Autodesk Inventor part; units mm, degrees
ref_plane "YZ Plane" through (0, 0, 0) normal (1, 0, 0) x (0, 1, 0)
ref_plane "XZ Plane" through (0, 0, 0) normal (0, 1, 0) x (-1, 0, 0)
ref_plane "XY Plane" through (0, 0, 0) normal (0, 0, 1) x (1, 0, 0)
sketch "bed" plane through (0, 0, 0) normal (0, 1, 0) x (-1, 0, 0)
  line L0 (59.3441, 94.0804) -> (59.3441, 91.0804)
  line L1 (59.3441, 91.0804) -> (91.3441, 91.0804)
  line L2 (-18.6559, 94.0804) -> (-18.6559, 91.0804)
  line L3 (-18.6559, 91.0804) -> (19.3441, 91.0804)
  line L4 (19.3441, 91.0804) -> (19.3441, 94.0804)
  line L5 (-18.6559, 94.0804) -> (-58.6559, 94.0804)
  line L6 (-58.6559, 94.0804) -> (-58.6559, 91.0804)
  line L7 (59.3441, 94.0804) -> (19.3441, 94.0804)
  line L8 (-58.6559, 91.0804) -> (-90.6559, 91.0804)
  line L9 (59.3441, -93.9196) -> (59.3441, -90.9196)
  line L10 (59.3441, -90.9196) -> (91.3441, -90.9196)
  line L11 (-18.6559, -93.9196) -> (-18.6559, -90.9196)
  line L12 (-18.6559, -90.9196) -> (19.3441, -90.9196)
  line L13 (-58.6559, -93.9196) -> (-58.6559, -90.9196)
  line L14 (59.3441, -93.9196) -> (19.3441, -93.9196)
  line L15 (-18.6559, -93.9196) -> (-58.6559, -93.9196)
  line L16 (-58.6559, -90.9196) -> (-90.6559, -90.9196)
  line L17 (94.3441, 59.0804) -> (91.3441, 59.0804)
  line L18 (94.3441, 59.0804) -> (94.3441, 19.0804)
  line L19 (91.3441, -18.9196) -> (91.3441, 19.0804)
  line L20 (94.3441, -18.9196) -> (91.3441, -18.9196)
  line L21 (94.3441, -58.9196) -> (91.3441, -58.9196)
  line L22 (94.3441, -18.9196) -> (94.3441, -58.9196)
  line L23 (91.3441, 59.0804) -> (91.3441, 91.0804)
  line L24 (91.3441, -58.9196) -> (91.3441, -90.9196)
  line L25 (84.2181, 86.0804) -> (-83.7819, 86.0804)
  line L26 (-85.7819, 84.0804) -> (-85.7819, -83.9196)
  line L27 (-83.7819, -85.9196) -> (84.2181, -85.9196)
  line L28 (86.2181, -83.9196) -> (86.2181, 84.0804)
  arc A0 (86.2181, 84.0804) -> (84.2181, 86.0804) centre (84.2181, 84.0804) ccw
  arc A1 (84.2181, -85.9196) -> (86.2181, -83.9196) centre (84.2181, -83.9196) ccw
  arc A2 (-85.7819, -83.9196) -> (-83.7819, -85.9196) centre (-83.7819, -83.9196) ccw
  arc A3 (-83.7819, 86.0804) -> (-85.7819, 84.0804) centre (-83.7819, 84.0804) ccw
  line L29 (-93.6559, -18.9196) -> (-93.6559, -58.9196)
  line L30 (-93.6559, -58.9196) -> (-90.6559, -58.9196)
  line L31 (-93.6559, -18.9196) -> (-90.6559, -18.9196)
  line L32 (-90.6559, -18.9196) -> (-90.6559, 19.0804)
  line L33 (-90.6559, 19.0804) -> (-93.6559, 19.0804)
  line L34 (-93.6559, 59.0804) -> (-90.6559, 59.0804)
  line L35 (-90.6559, 59.0804) -> (-90.6559, 91.0804)
  line L36 (-93.6559, 59.0804) -> (-93.6559, 19.0804)
  line L37 (-90.6559, -58.9196) -> (-90.6559, -90.9196)
  line L38 (19.3441, -90.9196) -> (19.3441, -93.9196)
  line L39 (91.3441, 19.0804) -> (94.3441, 19.0804)
  circle A4 centre (87.3441, -86.9196) radius 1.5
  circle A5 centre (87.3441, 87.0804) radius 1.5
  circle A6 centre (-86.6559, -86.9196) radius 1.5
  circle A7 centre (-86.6559, 87.0804) radius 1.5
  point P0 (-85.7819, -85.9196)
  point P1 (-85.7819, 86.0804)
  point P2 (86.2181, -85.9196)
  point P3 (-85.1961, 85.4946)
  point P4 (85.6323, 85.4946)
  dimension "d31" = 3
  dimension "d36" = 40
  dimension "d37" = 38
  dimension "d38" = 40
  dimension "d47" = 3
  dimension "d49" = 172
  dimension "d50" = 2
  dimension "d56" = 188
  dimension "d114" = 3
  dimension "d115" = 35
  dimension "d116" = 35
  dimension "d117" = 3
  dimension "d118" = 35
  dimension "d119" = 40
  dimension "d120" = 38
  dimension "d121" = 40
  dimension "d125" = 40
  dimension "d126" = 35
  dimension "d127" = 40
  dimension "d128" = 38
  dimension "d129" = 40
  dimension "d130" = 35
  dimension "d164" = 3
  dimension "d165" = 4
  dimension "d166" = 4
  dimension "d167" = 3
  dimension "d168" = 3
  dimension "d169" = 3
  dimension "d170" = 4
  dimension "d171" = 4
extrude "Extrusion1" add sketch "bed" along normal blind 3
sketch "Sketch10" plane through (93.6559, 0, 59.0804) normal (1, 0, 0) x (0, 0, -1)
  circle A0 centre (59, -13.7365) radius 1.5
  circle A1 centre (-15.1261, -13.7365) radius 1.5
  circle A2 centre (126.8739, -13.7365) radius 1.5
  line L0 (-32, 3) -> (0, 3)
  line L1 (0, 0) -> (0, 3)
  line L2 (0, 0) -> (40, 0)
  line L3 (40, 0) -> (40, 3)
  line L4 (40, 3) -> (78, 3)
  line L5 (78, 0) -> (78, 3)
  line L6 (78, 0) -> (118, 0)
  line L7 (118, 0) -> (118, 3)
  line L8 (118, 3) -> (150, 3)
  line L9 (-35, 3) -> (-32, 3)
  line L10 (-35, 3) -> (-35, -7)
  line L11 (-35, -7) -> (-32, -7)
  line L12 (-32, -7) -> (-32, -17)
  line L13 (150, -17) -> (150, -7)
  line L14 (150, -7) -> (153, -7)
  line L15 (150, 3) -> (153, 3)
  line L16 (153, -7) -> (153, 3)
  line L17 (-25, -25) -> (-25, -19)
  line L18 (-27, -17) -> (-32, -17)
  line L19 (143, -25) -> (143, -19)
  line L20 (145, -17) -> (150, -17)
  line L21 (-23, -27) -> (141, -27)
  arc A3 (-25, -19) -> (-27, -17) centre (-27, -19) ccw
  arc A4 (-25, -25) -> (-23, -27) centre (-23, -25) ccw
  arc A5 (141, -27) -> (143, -25) centre (141, -25) ccw
  arc A6 (145, -17) -> (143, -19) centre (145, -19) ccw
  point P0 (-25, -27)
  point P1 (-25, -17)
  point P2 (143, -17)
  point P3 (143, -27)
  dimension "d50" = 2
  dimension "d61" = 3
  dimension "d62" = 3
  dimension "d63" = 3
  dimension "d134" = 10
  dimension "d135" = 3
  dimension "d136" = 10
  dimension "d152" = 10
  dimension "d154" = 10
  dimension "d155" = 2
extrude "PRINT L" add sketch "Sketch10" against normal blind 3
sketch "Sketch13" plane through (-94.3441, 0, -58.9196) normal (-1, 0, 0) x (0, 0, 1)
  line L0 (-32, -7) -> (-32, -17)
  line L1 (-35, -7) -> (-32, -7)
  line L2 (-35, 3) -> (-35, -7)
  line L3 (150, -7) -> (153, -7)
  line L4 (153, -7) -> (153, 3)
  circle A0 centre (133.1261, -13.7365) radius 1.5
  circle A1 centre (59, -13.7365) radius 1.5
  circle A2 centre (-8.8739, -13.7365) radius 1.5
  line L5 (-35, 3) -> (-32, 3)
  line L6 (-32, 3) -> (0, 3)
  line L7 (0, 0) -> (0, 3)
  line L8 (0, 0) -> (40, 0)
  line L9 (40, 0) -> (40, 3)
  line L10 (40, 3) -> (78, 3)
  line L11 (78, 0) -> (78, 3)
  line L12 (78, 0) -> (118, 0)
  line L13 (118, 0) -> (118, 3)
  line L14 (118, 3) -> (150, 3)
  line L15 (150, 3) -> (153, 3)
  line L16 (-32, -17) -> (-27, -17)
  arc A3 (-25, -19) -> (-27, -17) centre (-27, -19) ccw
  line L17 (-25, -19) -> (-25, -25)
  arc A4 (-25, -25) -> (-23, -27) centre (-23, -25) ccw
  line L18 (-23, -27) -> (141, -27)
  arc A5 (141, -27) -> (143, -25) centre (141, -25) ccw
  line L19 (143, -25) -> (143, -19)
  arc A6 (145, -17) -> (143, -19) centre (145, -19) ccw
  line L20 (145, -17) -> (150, -17)
  line L21 (150, -17) -> (150, -7)
extrude "Right" add sketch "Sketch13" against normal blind 3
sketch "Sketch14" plane through (-59.3441, 0, 94.0804) normal (0, 0, 1) x (1, 0, 0)
  line L0 (-35, -7) -> (-32, -7)
  line L1 (-32, 3) -> (-32, -7)
  line L2 (-32, 3) -> (0, 3)
  line L3 (0, 0) -> (0, 3)
  line L4 (0, 0) -> (40, 0)
  line L5 (40, 0) -> (40, 3)
  line L6 (40, 3) -> (78, 3)
  line L7 (78, 0) -> (78, 3)
  line L8 (78, 0) -> (118, 0)
  line L9 (118, 3) -> (150, 3)
  line L10 (118, 0) -> (118, 3)
  line L11 (150, -7) -> (150, 3)
  line L12 (153, -7) -> (150, -7)
  circle A0 centre (59, -13.7365) radius 1.5
  circle A1 centre (-15.1261, -13.7365) radius 1.5
  circle A2 centre (126.8739, -13.7365) radius 1.5
  line L13 (-35, -17) -> (-35, -7)
  line L14 (153, -7) -> (153, -17)
  line L15 (-35, -17) -> (-27, -17)
  line L16 (-25, -19) -> (-25, -25)
  line L17 (153, -17) -> (145, -17)
  line L18 (143, -19) -> (143, -25)
  line L19 (-23, -27) -> (141, -27)
  arc A3 (-25, -25) -> (-23, -27) centre (-23, -25) ccw
  arc A4 (-25, -19) -> (-27, -17) centre (-27, -19) ccw
  arc A5 (145, -17) -> (143, -19) centre (145, -19) ccw
  arc A6 (141, -27) -> (143, -25) centre (141, -25) ccw
  point P0 (59.3441, 0)
  point P1 (-25, -27)
  point P2 (-25, -17)
  point P3 (143, -27)
  point P4 (143, -17)
  dimension "d50" = 2
  dimension "d144" = 3
  dimension "d145" = 3
  dimension "d146" = 3
  dimension "d157" = 10
  dimension "d159" = 10
  dimension "d160" = 2
extrude "PRINT UP" add sketch "Sketch14" against normal blind 3
sketch "Sketch15" plane through (58.6559, 0, -93.9196) normal (0, 0, -1) x (-1, 0, 0)
  circle A0 centre (-8.8739, -13.7365) radius 1.5
  circle A1 centre (59, -13.7365) radius 1.5
  circle A2 centre (133.1261, -13.7365) radius 1.5
  line L0 (-35, -7) -> (-32, -7)
  line L1 (-32, 3) -> (-32, -7)
  line L2 (-32, 3) -> (0, 3)
  line L3 (0, 0) -> (0, 3)
  line L4 (0, 0) -> (40, 0)
  line L5 (40, 0) -> (40, 3)
  line L6 (40, 3) -> (78, 3)
  line L7 (78, 0) -> (78, 3)
  line L8 (78, 0) -> (118, 0)
  line L9 (118, 0) -> (118, 3)
  line L10 (118, 3) -> (150, 3)
  line L11 (150, 0) -> (150, 3)
  line L12 (153, -7) -> (150, -7)
  line L13 (150, -7) -> (150, 3)
  line L14 (-35, -17) -> (-35, -7)
  line L15 (-35, -17) -> (-32, -17)
  line L16 (-32, -17) -> (-27, -17)
  arc A3 (-25, -19) -> (-27, -17) centre (-27, -19) ccw
  line L17 (-25, -19) -> (-25, -25)
  arc A4 (-25, -25) -> (-23, -27) centre (-23, -25) ccw
  line L18 (-23, -27) -> (141, -27)
  arc A5 (141, -27) -> (143, -25) centre (141, -25) ccw
  line L19 (143, -25) -> (143, -19)
  arc A6 (145, -17) -> (143, -19) centre (145, -19) ccw
  line L20 (145, -17) -> (150, -17)
  line L21 (153, -17) -> (150, -17)
  line L22 (153, -7) -> (153, -17)
  point P0 (58.6559, 0)
extrude "Down" add sketch "Sketch15" against normal blind 3
sketch "Sketch16" plane through (-94.3441, 3, 94.0804) normal (0, 1, 0) x (1, 0, 0)
  line L0 (188, 0) -> (0, 0)
  line L1 (188, 188) -> (188, 0)
  line L2 (188, 188) -> (185, 188)
  line L3 (3, 188) -> (185, 188)
  line L4 (0, 188) -> (3, 188)
  line L5 (0, 0) -> (0, 188)
  circle A0 centre (7, 181) radius 1.5
  circle A1 centre (7, 7) radius 1.5
  circle A2 centre (181, 181) radius 1.5
  circle A3 centre (181, 7) radius 1.5
  arc A4 (8.126, 10) -> (10.126, 8) centre (10.126, 10) ccw
  line L6 (8.126, 10) -> (8.126, 178)
  arc A5 (10.126, 180) -> (8.126, 178) centre (10.126, 178) ccw
  line L7 (10.126, 180) -> (178.126, 180)
  arc A6 (180.126, 178) -> (178.126, 180) centre (178.126, 178) ccw
  line L8 (180.126, 178) -> (180.126, 10)
  arc A7 (178.126, 8) -> (180.126, 10) centre (178.126, 10) ccw
  line L9 (178.126, 8) -> (10.126, 8)
  dimension "d50" = 2
extrude "Extrusion13" add sketch "Sketch16" along normal blind 3
properties part number "Bottom fabric holder" material "PET Plastic"
Check sheet for the modelled part. Datum: model origin and axes. Units: mm. A direction names the side the tool comes from. Round coordinates to 2 decimals unless told otherwise and drop trailing zeros. Loops run counter-clockwise (first coordinate to the right, second up) from the corner with the lowest first, then second, coordinate; pieces in that order, holes last. Notation, with made-up numbers: M 64,-28.75 L 91,-28.75 A31 cw 91,-3.75 Z; hole C -34,-5 d6. An arc over 180 degrees is marked long. Answer as a JSON object with one key per item and string values.
1. Access from +Z, -Z, +X, -X, +Y, -Y to the whole of each face (thin tool, end or side, straight path). Record for faces 5 (the flat face through (91, -17, -91)), 6 (the flat face through (-86.218, 3, 1)), 7 (the flat face through (90.656, -16, 1)).
Reply:
{"face 5": "-Z, +X, -Y", "face 6": "+Y, -Y", "face 7": "-Y"}
2. Gauge pin test, flat ends, axial feed: P1, Ø3.5, axis at x = 92.5, y = -21.5, coming from the +Z side; P2, Ø5, axis at x = 86.66, z = 87.08, coming from the -Y side; P3, Ø2.5, axis at y = -22, z = -92, coming from the +X side. Record the tip position at first contact, or that the pin passes through.
Reply:
{"P1": "stops at z = 84.08", "P2": "stops at y = 0", "P3": "stops at x = 83.66"}
3. Section check B-B (z = -28.5). Record the boundary of the cut face in (x, y).
Reply:
{"outline": "M -94.34,-27 L -91.34,-27 L -91.34,0 L -86.22,0 L -86.22,6 L -94.34,6 Z; M 85.78,0 L 90.66,0 L 90.66,-27 L 93.66,-27 L 93.66,6 L 85.78,6 Z"}
4. Scan lines: line 1 (X direction, y = -7.5, z = -2); line 2 (Z direction, x = 40.5, y = -25); line 3 (X direction, y = 4, z = -58.5). Record each from-to range of solid material in increasing order.
Reply:
{"line 1": "x = -94.34 to -91.34, 90.66 to 93.66", "line 2": "z = -93.92 to -90.92, 91.08 to 94.08", "line 3": "x = -94.34 to -86.22, 85.78 to 93.66"}
5. Section check A-A (x = -64). Record the boundary of the cut face in (y, z).
Reply:
{"outline": "M -27,-93.92 L 6,-93.92 L 6,-85.92 L 0,-85.92 L 0,-90.92 L -27,-90.92 Z; M -27,91.08 L 0,91.08 L 0,86.08 L 6,86.08 L 6,94.08 L -27,94.08 Z"}
6. Mould release check, pull along X, two halves, no side actions. Record for faces 1 (the flat face through (-91.344, -16, -1)), 2 (the flat face through (91, -17, 92)), 3 (the flat face through (93.656, -11, -1)), 4 (the flat face through (-2, -16, 91.08)): pulls with the +X half, pulls with the -X half, needs draft (parallel to the pull), parting line crosses it, or undercut.
Reply:
{"face 1": "undercut", "face 2": "needs draft", "face 3": "pulls with the +X half", "face 4": "undercut"}
